Work out the finished part from the listing and answer in its coordinate system (mm). A direction names the side the tool comes from. Round coordinates to 2 decimals unless told otherwise and drop trailing zeros. Write each loop counter-clockwise with the first axis right and the second up, starting at its lowest first coordinate (ties: lowest second). Pieces come first, ordered by that corner, then holes.
1. Find section B-B (z = -15). Write down the section's boundary in (x, y).
2. A tool of negligible diameter and unlimited length cuts with its end or side. For faces 4 (the face through (-14.125, 5.856, 75.776)), 5 (the face through (-3.94, -2.28, -33.147)), 6 (the face through (-7.43, 7.48, 76.04)), 7 (the face through (-1.34, -10.23, -15.99)), 8 (the face through (8.585, 0, -31)), from which of +Z, -Z, +X, -X, +Y, -Y can it reach the whole face along a straight path? Write none if from no direction.
3. Flat-ended cylindrical pins translate along their axes: pin 1 Ø8 at (y, z) = (-5, 26.5) entering from +X; pin 2 Ø6 at (x, y) = (0, 0) entering from -Z; pin 3 Ø1.5 at (y, z) = (3.5, 54) entering from +X. Find the tip coordinate at first contact, or state that the pin passes through.
4. Find section A-A (z = 52). Write down the section's boundary in (x, y), and give its area (3 significant figures).
5. Determine the mould class of faces 1 (the face through (0, 0, 68.199)), 2 (the face through (-8.585, 0, -31)), 3 (the face through (15.77, 4.97, 35.16)) for opening direction X: pulls with the +X half, pulls with the -X half, needs draft (parallel to the pull), parting line crosses it, or undercut.
6. Straight lines are drawn through the part: probe 1 along Y at (x, z) = (0, -22); probe 2 along Y at (x, z) = (-0.5, 74); probe 3 along Z at (x, y) = (1, -12). For each, find the intervals that lie inside material, in ascending order.
```python
from build123d import *

# Parameters (mm, degrees)
SKETCH1_R          = 16.5354
EXTRUDE1_DEPTH     = 82.423
CHAMFER1_SIZE      = 0.762
SKETCH6_R          = 15.6845
EXTRUDE2_DEPTH     = 5.969
SKETCH7_W          = 27.178
SKETCH7_H          = 10.31875
CUT_EXTRUDE4_DEPTH = 19.84248
HOLE1_D            = 5.0038
HOLE1_DEPTH        = 4.7498
CIRPATTERN1_COUNT  = 4


with BuildPart() as part:
    # Sketch1 → Extrude1 (new body)
    with BuildSketch(Plane.XY):
        Circle(SKETCH1_R)
    extrude(amount=EXTRUDE1_DEPTH)

    # Sketch2 → Cut-Revolve1 (revolve, cut)
    with BuildSketch(Plane(origin=(0, 0, 0), x_dir=(1, 0, 0), z_dir=(0, 1, 0)), mode=Mode.PRIVATE) as cut_revolve1_sk:
        Polygon((16.5354, -82.423), (16.5354, -68.4784), (15.2908, -69.723), (15.2908, -82.423), align=None)
    revolve(cut_revolve1_sk.sketch.rotate(Axis((0, 0, 0), (0, 0, 1)), 180), axis=Axis((0, 0, 0), (0, 0, 1)), mode=Mode.SUBTRACT)  # turned: the seam where the file's is

    # Sketch3 → Cut-Revolve2 (revolve, cut)
    with BuildSketch(Plane(origin=(0, 0, 0), x_dir=(1, 0, 0), z_dir=(0, 1, 0)), mode=Mode.PRIVATE) as cut_revolve2_sk:
        Polygon((15.2908, 0), (15.2908, -1.524), (16.5354, -2.7686), (16.5354, 0), align=None)
    revolve(cut_revolve2_sk.sketch.rotate(Axis((0, 0, 0), (0, 0, -1)), 180), axis=Axis((0, 0, 0), (0, 0, -1)), mode=Mode.SUBTRACT)  # turned: the seam where the file's is

    # S2D0002 → Cut-Revolve3 (revolve, cut)
    with BuildSketch(Plane(origin=(0, 0, 0), x_dir=(1, 0, 0), z_dir=(0, 1, 0))):
        Polygon((6.1849, -82.169), (9.525, -82.169), (9.525, -82.423), (0, -82.423), (0, -68.199), (4.9784, -68.199), (4.9784, -78.952393135), (5.642306865, -79.6163), align=None)
    revolve(axis=Axis((0, 0, 14.6685), (0, 0, -1)), mode=Mode.SUBTRACT)

    # Chamfer1
    chamfer1_edges = [part.edges().sort_by_distance(p)[0] for p in [
        (15.2908, 0, 82.423),
    ]]
    chamfer(chamfer1_edges, length=CHAMFER1_SIZE)

    # Sketch6 → Extrude2 (add)
    with BuildSketch(Plane(origin=(0, 0, 0), x_dir=(-1, 0, 0), z_dir=(0, 0, -1))):
        Circle(SKETCH6_R)
    extrude(amount=EXTRUDE2_DEPTH)

    # Sketch7 → Revolve1 (revolve)
    with BuildSketch(Plane(origin=(0, 0, 0), x_dir=(0, 0, -1), z_dir=(1, 0, 0)), mode=Mode.PRIVATE) as revolve1_sk:
        with Locations((19.558, -5.159375)):
            Rectangle(SKETCH7_W, SKETCH7_H)
    revolve(revolve1_sk.sketch.rotate(Axis((0, 0, 0), (0, 0, -1)), 270), axis=Axis((0, 0, 0), (0, 0, -1)))  # turned: the seam where the file's is

    # S2D0001 → Cut-Revolve5 (revolve, cut)
    with BuildSketch(Plane(origin=(0, 0, 0), x_dir=(1, 0, 0), z_dir=(0, 1, 0))):
        Polygon((3.2639, 31.211260017), (3.2639, 18.2118), (0, 18.2118), (0, 33.147), (4.3815, 33.147), align=None)
    revolve(axis=Axis((0, 0, 31.308359971), (0, 0, -1)), mode=Mode.SUBTRACT)

    # Sketch9 → Cut-Revolve6 (revolve, cut)
    with BuildSketch(Plane(origin=(0, 0, 0), x_dir=(0, -1, 0), z_dir=(1, 0, 0)), mode=Mode.PRIVATE) as cut_revolve6_sk:
        with BuildLine():
            Line((-10.31875, 25.7302), (-10.033, 26.4922))
            Line((-10.033, 26.4922), (-10.033, 32.131))
            ThreePointArc((-10.033, 32.131), (-9.932678675, 32.674796865), (-9.644922533, 33.147))
            Line((-9.644922533, 33.147), (-10.31875, 33.147))
            Line((-10.31875, 33.147), (-10.31875, 25.7302))
        make_face()
    revolve(cut_revolve6_sk.sketch.rotate(Axis((0, 0, -12.65936), (0, 0, -1)), 90), axis=Axis((0, 0, -12.65936), (0, 0, -1)), mode=Mode.SUBTRACT)  # turned: the seam where the file's is

    # Sketch13 → Cut-Extrude4 (cut, symmetric)
    with BuildSketch(Plane(origin=(0, 0, 0), x_dir=(1, 0, 0), z_dir=(0, 1, 0))):
        Polygon((8.5852, 33.147), (8.5852, 28.194), (10.033, 26.7462), (10.033, 33.147), align=None)
        Polygon((-8.5852, 33.147), (-8.5852, 28.194), (-10.033, 26.7462), (-10.033, 33.147), align=None)
    extrude(amount=CUT_EXTRUDE4_DEPTH, both=True, mode=Mode.SUBTRACT)

    # Hole1
    with Locations(Plane(origin=(-10.81222837, 10.81222837, 76.073), x_dir=(0.707106781, 0.707106781, 0), z_dir=(-0.707106781, 0.707106781, 0))):
        with Locations((0, 0)):
            hole1 = Hole(HOLE1_D / 2, depth=HOLE1_DEPTH)

    # CirPattern1: Hole1 ×4 about axis
    cirpattern1_axis = Axis((0, 0, 0), (0, 0, 1))
    for i in range(1, CIRPATTERN1_COUNT):
        add(hole1.rotate(cirpattern1_axis, i * 360 / CIRPATTERN1_COUNT), mode=Mode.SUBTRACT)


solid = part.part
```
Worked answers:
1. outline: circle Ø20.64 at (0, 0)
2. face 4: +Z
2. face 5: -Z, +X, -X, +Y, -Y
2. face 6: none
2. face 7: -Z
2. face 8: -Z, +X, +Y, -Y
3. pin 1: stops at x = 16.51
3. pin 2: stops at z = -18.21
3. pin 3: stops at x = 16.31
4. outline: circle Ø33.07 at (0, 0)
4. area: 859 mm2
5. face 1: undercut
5. face 2: pulls with the -X half
5. face 3: parting line crosses it
6. probe 1: y = -10.32 to -3.26, 3.26 to 10.32
6. probe 2: y = -15.28 to -4.95, 4.95 to 15.28
6. probe 3: z = -5.97 to 82.42
